from build123d import *

# Parameters (mm, degrees)
SKETCH_1_R          = 9
EXTRUDE_1_DEPTH     = 8
SKETCH_3_R          = 6.5
EXTRUDE_2_DEPTH     = 8
EXTRUDE_3_DEPTH     = 6
SKETCH_5_R          = 6.5
EXTRUDE_4_DEPTH     = 11
SKETCH_8_R          = 6.5
CUT_EXTRUDE_3_DEPTH = 11
SKETCH_9_W          = 1.361349768
SKETCH_9_H          = 3
SKETCH_10_R         = 4.5
CUT_EXTRUDE_4_DEPTH = 29.906458333


# Read off the part's stored shape, not the designer's step: M18 机械螺纹 螺柱1, G1/8 直管螺纹 螺柱1
with BuildPart() as part:
    # 草图1 → 凸台-拉伸1 (new body)
    with BuildSketch(Plane.XY):
        Circle(SKETCH_1_R)
    extrude(amount=-EXTRUDE_1_DEPTH)

    # 草图3 → 凸台-拉伸2 (add)
    with BuildSketch(Plane.XY):
        Circle(SKETCH_3_R)
    extrude(amount=-EXTRUDE_2_DEPTH)

    # 草图4 → 凸台-拉伸3 (add)
    with BuildSketch(Plane(origin=(0, 0, -8), x_dir=(-1, 0, 0), z_dir=(0, 0, -1))):
        Polygon((0, 10.969655115), (-9.5, 5.484827557), (-9.5, -5.484827557), (0, -10.969655115), (9.5, -5.484827557), (9.5, 5.484827557), align=None)
    extrude(amount=EXTRUDE_3_DEPTH)

    # 草图5 → 凸台-拉伸4 (add)
    with BuildSketch(Plane(origin=(0, 0, -14), x_dir=(-1, 0, 0), z_dir=(0, 0, -1))):
        with Locations(Location((0, 0, 0), (0, 0, 180))):
            Circle(SKETCH_5_R)
    extrude(amount=EXTRUDE_4_DEPTH)

    # M18 机械螺纹 螺柱1 outline → M18 机械螺纹 螺柱1 (revolve, cut)
    with BuildSketch(Plane.XZ):
        Polygon((9, 0), (7.647, 0), (9, -1.353), align=None)
    revolve(axis=Axis((0, 0, 0), (0, 0, 1)), mode=Mode.SUBTRACT)

    # G1/8 直管螺纹 螺柱1 outline → G1/8 直管螺纹 螺柱1 (revolve, cut)
    with BuildSketch(Plane.XZ):
        Polygon((6.5, -14), (4.864, -14), (4.864, -24.419), (4.283, -25), (6.5, -25), align=None)
    revolve(axis=Axis((0, 0, 0), (0, 0, 1)), mode=Mode.SUBTRACT)

    # 草图8 → 切除-拉伸3 (cut)
    with BuildSketch(Plane.XY):
        Circle(SKETCH_8_R)
    extrude(amount=-CUT_EXTRUDE_3_DEPTH, mode=Mode.SUBTRACT)

    # 草图9 → 切除-旋转1 (revolve, cut)
    with BuildSketch(Plane(origin=(0, 0, 0), x_dir=(1, 0, 0), z_dir=(0, 1, 0)), mode=Mode.PRIVATE) as cut_revolve_1_sk:
        with Locations((8.319325116, 6.5)):
            Rectangle(SKETCH_9_W, SKETCH_9_H)
    revolve(cut_revolve_1_sk.sketch.rotate(Axis((0, 0, -7.326856085), (0, 0, 1)), 180), axis=Axis((0, 0, -7.326856085), (0, 0, 1)), mode=Mode.SUBTRACT)

    # 草图10 → 切除-拉伸4 (cut, through all)
    with BuildSketch(Plane(origin=(0, 0, -25), x_dir=(-1, 0, 0), z_dir=(0, 0, -1))):
        with Locations(Location((0, 0, 0), (0, 0, 180))):
            Circle(SKETCH_10_R)
    extrude(amount=-CUT_EXTRUDE_4_DEPTH, mode=Mode.SUBTRACT)


solid = part.part
Could you check a few things on this model? Use its own coordinates, in mm. A direction names the side the tool comes from. Give positions to 0.01 mm unless a question says otherwise; leave off trailing zeros. Loops run counter-clockwise (first coordinate to the right, second up) from the corner with the lowest first, then second, coordinate; pieces in that order, holes last. Notation, with made-up numbers: (5, 89.25) -> (25, 89.25) arc R11 cw to (25, 106.25) -> close; hole circle Ø7 at (11, -28). An arc over 180 degrees is marked (long way). Return JSON: item names as keys, results as strings.
Item 1: If we section it at B-B on z = -13: List the corners of the cut face in (x, y) for me, plus the area to 3 significant figures.
Geometry results:
{"outline": "(-9.5, -5.48) -> (0, -10.97) -> (9.5, -5.48) -> (9.5, 5.48) -> (0, 10.97) -> (-9.5, 5.48) -> close; hole circle Ø9 at (0, 0)", "area": "249 mm²"}
Item 2: If we section it at D-D on z = -2.5: List the corners of the cut face in (x, y) for me.
Geometry results:
{"outline": "circle Ø18 at (0, 0); hole circle Ø13 at (0, 0)"}
Item 3: If we section it at C-C on z = -8.75: List the corners of the cut face in (x, y) for me.
Geometry results:
{"outline": "(-9.5, -5.48) -> (0, -10.97) -> (9.5, -5.48) -> (9.5, 5.48) -> (0, 10.97) -> (-9.5, 5.48) -> close; hole circle Ø13 at (0, 0)"}
Item 4: I need wall thicknesses on L1, parallel to Y at x = 0, z = -4; L2, parallel to Z at x = 8.75, y = -5.75; L3, parallel to Z at x = 6, y = -1.5. Which ranges of each line are inside material? Lowest first, please. Write a range as from..to.
Geometry results:
{"L1": "y = -9..-6.5, 6.5..9", "L2": "z = -14..-8", "L3": "z = -14..-11"}
Item 5: Which directions (+Z, -Z, +X, -X, +Y, -Y) give clear straight access to the entire face, cutting with the end or side of a thin tool? Please do faces 1 (the flat face through (-4, 7, -5)), 2 (the cylindrical face through (4.64, 1.46, -19.28)), 3 (the cylindrical face through (-1.172, 8.923, -3.151)).
Geometry results:
{"face 1": "none", "face 2": "-Z", "face 3": "+Z"}
Item 6: I'm going to push flat-ended pins straight in: pin 1 (1.5 mm diameter, centred on y = 6, z = -19, fed in from -X); pin 2 (1 mm diameter, centred on x = 4.5, z = -4.5, fed in from -Y); pin 3 (8 mm diameter, centred on x = -3.5, z = -11, fed in from -Y); pin 4 (1 mm diameter, centred on x = 1.5, z = -5, fed in from -Y). Where does each tip first touch, or does it pass through?
Geometry results:
{"pin 1": "passes through", "pin 2": "stops at y = -8.06", "pin 3": "stops at y = -10.97", "pin 4": "stops at y = -8.94"}
Item 7: If we section it at A-A on y = 0: List the corners of the cut face in (x, z) for me, plus the area to 3 significant figures.
Geometry results:
{"outline": "(-9.5, -14) -> (-4.86, -14) -> (-4.86, -24.42) -> (-4.5, -24.78) -> (-4.5, -11) -> (-6.5, -11) -> (-6.5, 0) -> (-7.65, 0) -> (-9, -1.35) -> (-9, -5) -> (-7.64, -5) -> (-7.64, -8) -> (-9.5, -8) -> close; (4.5, -24.78) -> (4.86, -24.42) -> (4.86, -14) -> (9.5, -14) -> (9.5, -8) -> (7.64, -8) -> (7.64, -5) -> (9, -5) -> (9, -1.35) -> (7.65, 0) -> (6.5, 0) -> (6.5, -11) -> (4.5, -11) -> close", "area": "85.7 mm²"}
Item 8: We'd pull the mould along X, two halves only. Please class faces 4 (the flat face through (-4.42, 1.54, -11)), 5 (the flat face through (2, -5, -14)), 6 (the flat face through (9.5, 0, -11)): +X half, -X half, draft (parallel to the pull), parting line (faces both ways), or undercut.
Geometry results:
{"face 4": "undercut", "face 5": "draft", "face 6": "+X half"}
